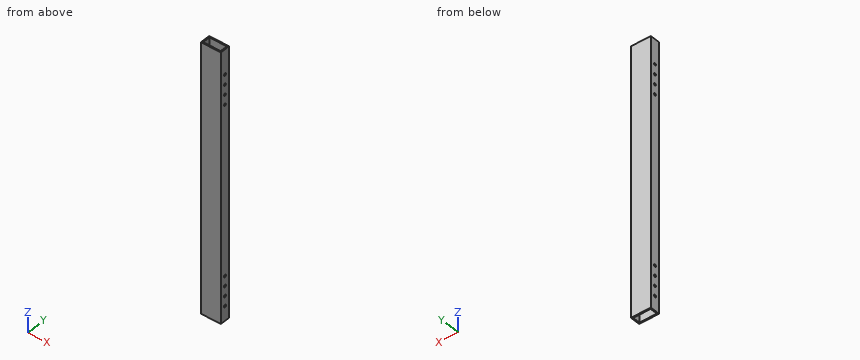
```python
from build123d import *

# Parameters (mm, degrees)
BOSS_EXTRUDE1_DEPTH         = 342.9
BOSS_EXTRUDE1_DEPTH_BACK    = 342.9
SKETCH3_W                   = 50.8
SKETCH3_H                   = 25.4
SKETCH3_W_2                 = 44.45
SKETCH3_H_2                 = 19.05
A_0_234_DIAMETER_HOLE1_D    = 5.9436
F_1_4_0_25_DIAMETER_HOLE2_D = 6.35


with BuildPart() as part:
    # Sketch3 → Boss-Extrude1 (new, two sides: drawn at the far end of the back side and taken through both)
    with BuildSketch(Plane.XY.offset(-BOSS_EXTRUDE1_DEPTH_BACK)):
        Rectangle(SKETCH3_W, SKETCH3_H)
        Rectangle(SKETCH3_W_2, SKETCH3_H_2, mode=Mode.SUBTRACT)
    extrude(amount=BOSS_EXTRUDE1_DEPTH + BOSS_EXTRUDE1_DEPTH_BACK)

    # A (0.234) Diameter Hole1 (through all)
    with Locations(Plane(origin=(25.4, 0, 0), x_dir=(0, 0, -1), z_dir=(1, 0, 0))):
        with Locations((-279.4, 0), (-254, 0), (-228.6, 0), (-203.2, 0)):
            Hole(A_0_234_DIAMETER_HOLE1_D / 2)

    # 1/4 (0.25) Diameter Hole2 (through all)
    with Locations(Plane(origin=(25.4, 0, 0), x_dir=(0, 0, -1), z_dir=(1, 0, 0))):
        with Locations((305.511799988, 0), (280.111799988, 0), (254.711799988, 0), (229.311799988, 0)):
            Hole(F_1_4_0_25_DIAMETER_HOLE2_D / 2)


solid = part.part
```
Check sheet for the modelled part. Datum: model origin and axes. Units: mm. Coordinates: 2 decimals unless noted, no trailing zeros. Order: outer loops, then holes, each group sorted by start corner. A loop starts at its lowest first (then second) coordinate and runs counter-clockwise, first axis right, second up. Notation, with made-up numbers: (27, 5.25) -> (63, 5.25) arc R29 ccw to (63, 38.25) -> close; hole circle Ø7 at (56, -29.5). An arc over 180 degrees is marked (long way). Write item = value, one per line. Start each with the question number.
1) Cross-section at B-B (x = -8). Enter the section's corners in (y, z) (3 decimals).
2) Material ranges on L1, parallel to Y at x = -16.5, z = -5 (3 decimals); L2, parallel to X at y = 1.75, z = 183.5 (3 decimals); L3, parallel to Y at x = 24, z = 279, recorded low to high.
3) Cross-section at A-A (z = 81). Enter the section's corners in (x, y) (3 decimals), then the cut area to 3 significant figures.
Ans:
q1.outline = (-12.7, -342.9) -> (-9.525, -342.9) -> (-9.525, 342.9) -> (-12.7, 342.9) -> close; (9.525, -342.9) -> (12.7, -342.9) -> (12.7, 342.9) -> (9.525, 342.9) -> close
q2.L1 = -12.7 to -9.525, 9.525 to 12.7
q2.L2 = -25.4 to -22.225, 22.225 to 25.4
q2.L3 = -12.7 to -2.94, 2.94 to 12.7
q3.outline = (-25.4, -12.7) -> (25.4, -12.7) -> (25.4, 12.7) -> (-25.4, 12.7) -> close; hole (-22.225, -9.525) -> (22.225, -9.525) -> (22.225, 9.525) -> (-22.225, 9.525) -> close
q3.area = 444 mm²
